The listing builds one solid part. Answer for the finished solid, in the listing's coordinates (mm). A direction names the side the tool comes from. Round coordinates to 2 decimals unless told otherwise and drop trailing zeros. Write each loop counter-clockwise with the first axis right and the second up, starting at its lowest first coordinate (ties: lowest second). Pieces come first, ordered by that corner, then holes.
Item 1: Find the intervals of material crossed by probe 1 along Y at (x, z) = (-0.75, -3.5); probe 2 along X at (y, z) = (5.75, -13.75) (3 decimals); probe 3 along Y at (x, z) = (-0.75, -6.75), in increasing order.
Item 2: Find section B-B on z = -15. Give the vertices of the cut face in (x, y), then the cut area to 3 significant figures.
Item 3: Each of these flat-tipped pins is pushed along its axis until it touches: pin 1 (2 mm diameter, centred on x = 5, z = -11, fed in from +Y); pin 2 (3 mm diameter, centred on y = 3, z = -2.5, fed in from -X) (3 decimals); pin 3 (6.5 mm diameter, centred on x = -2, z = 0.5, fed in from +Y) (3 decimals). Where does it stop, or does it pass through?
Item 4: Find section A-A on y = 0. Give the vertices of the cut face in (x, z) (3 decimals).
Item 5: For a pull along Z with two mould halves and no side action, classify faces 1 (the face through (2, -6.58, -14)), 2 (the face through (-5.9, 0, -2.4)), 3 (the face through (2, -8, -14.3)) as +Z half, -Z half, draft (parallel to the pull), parting line (faces both ways), or undercut.
Item 6: Find section D-D on x = 1.75. Give the number of separate pieces and of enclosed holes in the cut face, then the cut area to 3 significant figures.
Item 7: Find section C-C on x = -4.75. Give the vertices of the cut face in (y, z) (3 decimals).
Item 8: A tool of negligible diameter and unlimited length cuts with its end or side. For faces 4 (the face through (3.483, -3, -14)), 5 (the face through (2.525, 9, -7)), 6 (the face through (6.275, 0, -7)), 7 (the face through (-4, 7.35, -14)), 8 (the face through (-2, -9.22, -10)), from which of +Z, -Z, +X, -X, +Y, -Y can it reach the whole face along a straight path? Write none if from no direction.
```python
from build123d import *

# Parameters (mm, degrees)
SKETCH1_W                = 14.95
SKETCH1_H                = 20.95
SKETCH1_W_2              = 11
SKETCH1_H_2              = 16
BOSS_EXTRUDE1_DEPTH      = 2
SKETCH2_W                = 12.55
SKETCH2_H                = 17.3
BOSS_EXTRUDE2_DEPTH      = 13.3
SKETCH3_W                = 6.2
SKETCH3_H                = 18.44
BOSS_EXTRUDE3_DEPTH      = 8.8
BOSS_EXTRUDE4_DEPTH      = 2.525
BOSS_EXTRUDE4_DEPTH_BACK = 2.5
BOSS_EXTRUDE5_DEPTH      = 7.14
SKETCH6_W                = 2.5
SKETCH6_H                = 2
BOSS_EXTRUDE6_DEPTH      = 1
CUT_EXTRUDE1_DEPTH       = 12.55
SKETCH8_W                = 11
SKETCH8_H                = 16
CUT_EXTRUDE2_DEPTH       = 4
FILLET1_R                = 0.5


with BuildPart() as part:
    # Sketch1 → Boss-Extrude1 (new body)
    with BuildSketch(Plane.XY):
        Rectangle(SKETCH1_W, SKETCH1_H)
        Rectangle(SKETCH1_W_2, SKETCH1_H_2, mode=Mode.SUBTRACT)
    extrude(amount=BOSS_EXTRUDE1_DEPTH)

    # Sketch2 → Boss-Extrude2 (add)
    with BuildSketch(Plane(origin=(0, 0, 0), x_dir=(-1, 0, 0), z_dir=(0, 0, -1))):
        Rectangle(SKETCH2_W, SKETCH2_H)
    extrude(amount=BOSS_EXTRUDE2_DEPTH)

    # Sketch3 → Boss-Extrude3 (add)
    with BuildSketch(Plane.ZY.offset(6.275)):
        with Locations((-10.2, 0)):
            Rectangle(SKETCH3_W, SKETCH3_H)
    extrude(amount=-BOSS_EXTRUDE3_DEPTH)

    # Sketch4 → Boss-Extrude4 (add, two sides)
    with BuildSketch(Plane(origin=(0, 0, 0), x_dir=(0, 0, -1), z_dir=(1, 0, 0))) as boss_extrude4_sk:
        Polygon((7.1, -9.22), (4, -10.65), (3.35, -10.65), (3.35, -10.3705), (2.7, -10.3705), (2.7, -10.23075), (2.05, -10.23075), (2.05, -10.091), (1.4, -10.091), (1.4, -9.95125), (0.75, -9.95125), (0.75, -9.8115), (0, -9.8115), (0, -9.22), (4, -10.08), (7.1, -8.65), align=None)
        Polygon((7.1, 9.22), (7.1, 8.65), (4, 10.08), (0, 9.22), (0, 9.8115), (0.75, 9.8115), (0.75, 9.95125), (1.4, 9.95125), (1.4, 10.091), (2.05, 10.091), (2.05, 10.23075), (2.7, 10.23075), (2.7, 10.3705), (3.35, 10.3705), (3.35, 10.65), (4, 10.65), align=None)
    extrude(amount=BOSS_EXTRUDE4_DEPTH)
    extrude(boss_extrude4_sk.sketch, amount=-BOSS_EXTRUDE4_DEPTH_BACK)

    # Sketch5 → Boss-Extrude5 (add)
    with BuildSketch(Plane(origin=(0, 0, -13.3), x_dir=(-1, 0, 0), z_dir=(0, 0, -1))):
        Polygon((0.5, 6.35), (-0.5, 6.35), (-0.5, -0.58), (-6, -0.58), (-6, -1.58), (-0.5, -1.58), (-0.5, -8.65), (0.5, -8.65), (0.5, -1.58), (6, -1.58), (6, -0.58), (0.5, -0.58), align=None)
    extrude(amount=BOSS_EXTRUDE5_DEPTH)

    # Sketch6 → Boss-Extrude6 (add)
    with BuildSketch(Plane(origin=(0, 0, -13.3), x_dir=(-1, 0, 0), z_dir=(0, 0, -1))):
        with Locations((2.232930788, -2.58)):
            Rectangle(SKETCH6_W, SKETCH6_H)
        with Locations((2.232930788, -7.58)):
            Rectangle(SKETCH6_W, SKETCH6_H)
        with Locations((-2.232930788, -7.58)):
            Rectangle(SKETCH6_W, SKETCH6_H)
        with Locations((-2.232930788, -2.58)):
            Rectangle(SKETCH6_W, SKETCH6_H)
        with Locations((4.275, 6.35)):
            Rectangle(SKETCH6_W, SKETCH6_H)
        with Locations((-4.275, 6.35)):
            Rectangle(SKETCH6_W, SKETCH6_H)
    extrude(amount=BOSS_EXTRUDE6_DEPTH)

    # Sketch7 → Cut-Extrude1 (cut)
    with BuildSketch(Plane(origin=(6.275, 0, 0), x_dir=(0, 0, -1), z_dir=(1, 0, 0))):
        with BuildLine():
            Line((1.2, 1.2), (0, 1.2))
            Line((0, 1.2), (0, -1.2))
            Line((0, -1.2), (1.2, -1.2))
            ThreePointArc((1.2, -1.2), (2.4, 0), (1.2, 1.2))
        make_face()
    extrude(amount=-CUT_EXTRUDE1_DEPTH, mode=Mode.SUBTRACT)

    # Sketch8 → Cut-Extrude2 (cut)
    with BuildSketch(Plane.XY):
        Rectangle(SKETCH8_W, SKETCH8_H)
    extrude(amount=-CUT_EXTRUDE2_DEPTH, mode=Mode.SUBTRACT)

    # Fillet1
    fillet1_edges = [part.edges().sort_by_distance(p)[0] for p in [
        (-7.475, 10.475, 1),
        (7.475, 10.475, 1),
        (7.475, -10.475, 1),
        (-7.475, -10.475, 1),
    ]]
    fillet(fillet1_edges, radius=FILLET1_R)


solid = part.part
```
Check values:
1. probe 1: y = -10.65 to -9.97, -8.65 to -8, 8 to 8.65, 9.97 to 10.65
1. probe 2: x = -5.525 to -3.025, -0.5 to 0.5, 3.025 to 5.525
1. probe 3: y = -9.38 to -8.81, -8.65 to 8.65, 8.81 to 9.38
2. outline: (-6, -1.58) - (-0.5, -1.58) - (-0.5, -8.65) - (0.5, -8.65) - (0.5, -1.58) - (6, -1.58) - (6, -0.58) - (0.5, -0.58) - (0.5, 6.35) - (-0.5, 6.35) - (-0.5, -0.58) - (-6, -0.58) - close
2. area: 26.0 mm2
3. pin 1: stops at y = 8.65
3. pin 2: stops at x = -6.275
3. pin 3: stops at y = 10.475
4. outline: (-7.475, 0) - (-5.5, 0) - (-5.5, 2) - (-7.475, 2) - close; (-6.275, -13.3) - (-0.5, -13.3) - (-0.5, -20.44) - (0.5, -20.44) - (0.5, -13.3) - (6.275, -13.3) - (6.275, -2.4) - (5.5, -2.4) - (5.5, -4) - (-5.5, -4) - (-5.5, -2.4) - (-6.275, -2.4) - close; (5.5, 0) - (7.475, 0) - (7.475, 2) - (5.5, 2) - close
5. face 1: draft
5. face 2: undercut
5. face 3: -Z half
6. separate pieces: 1
6. enclosed holes: 2
6. area: 202 mm2
7. outline: (-10.475, 0) - (-8.65, 0) - (-8.65, -7.1) - (-9.22, -7.1) - (-9.22, -13.3) - (-1.58, -13.3) - (-1.58, -20.44) - (-0.58, -20.44) - (-0.58, -13.3) - (5.35, -13.3) - (5.35, -14.3) - (7.35, -14.3) - (7.35, -13.3) - (9.22, -13.3) - (9.22, -7.1) - (8.65, -7.1) - (8.65, 0) - (10.475, 0) - (10.475, 2) - (8, 2) - (8, -4) - (-8, -4) - (-8, 2) - (-10.475, 2) - close
8. face 4: -Z, +X, -Y
8. face 5: -Z, +X, +Y
8. face 6: -Z, +X, +Y, -Y
8. face 7: -Z, +X, -X, +Y
8. face 8: -Z, +X, -X, -Y
